```python
from build123d import *

# Parameters (mm, degrees)
SK_MAIN_EXTRUSION_R   = 3.4
SK_MAIN_EXTRUSION_R_2 = 9
MAIN_EXTRUSION_DEPTH  = 25


with BuildPart() as part:
    # Sk Main Extrusion → Main Extrusion (new body)
    with BuildSketch(Plane.XY):
        with BuildLine():
            Line((-35.964339765, 8.84120158), (-38.698942589, 10.116367819))
            ThreePointArc((-38.698942589, 10.116367819), (-39.146142418, 10.175242794), (-39.546236371, 9.966967065))
            Line((-39.546236371, 9.966967065), (-48.436814511, 1.076388924))
            ThreePointArc((-48.436814511, 1.076388924), (-48.876154339, 0.015728753), (-48.436814511, -1.044931419))
            Line((-48.436814511, -1.044931419), (-35.355339059, -14.126406871))
            ThreePointArc((-35.355339059, -14.126406871), (0, -28.771067812), (35.355339059, -14.126406871))
            Line((35.355339059, -14.126406871), (48.436814511, -1.044931419))
            ThreePointArc((48.436814511, -1.044931419), (48.876154339, 0.015728753), (48.436814511, 1.076388924))
            Line((48.436814511, 1.076388924), (39.546236371, 9.966967065))
            ThreePointArc((39.546236371, 9.966967065), (39.146142418, 10.175242794), (38.698942589, 10.116367819))
            Line((38.698942589, 10.116367819), (35.964339765, 8.84120158))
            ThreePointArc((35.964339765, 8.84120158), (35.87848322, 8.775321536), (35.828512874, 8.679329395))
            Line((35.828512874, 8.679329395), (35.425239457, 7.174292513))
            Line((35.425239457, 7.174292513), (35.753978107, 6.469310204))
            Line((35.753978107, 6.469310204), (38.336524222, 5.265049173))
            ThreePointArc((38.336524222, 5.265049173), (38.606308031, 4.948092133), (38.542703923, 4.53675336))
            ThreePointArc((38.542703923, 4.53675336), (36.486225813, 2.654969004), (33.783331243, 1.973371234))
            Line((33.783331243, 1.973371234), (32.420845917, 1.973371234))
            ThreePointArc((32.420845917, 1.973371234), (25.880108191, 4.682633508), (23.170845917, 11.223371234))
            Line((23.170845917, 11.223371234), (23.170845917, 12.585856559))
            ThreePointArc((23.170845917, 12.585856559), (23.852443688, 15.28875113), (25.734228043, 17.34522924))
            ThreePointArc((25.734228043, 17.34522924), (26.145566816, 17.408833348), (26.462523856, 17.139049539))
            Line((26.462523856, 17.139049539), (27.666784887, 14.556503424))
            Line((27.666784887, 14.556503424), (28.371767196, 14.227764774))
            Line((28.371767196, 14.227764774), (29.876804078, 14.631038191))
            ThreePointArc((29.876804078, 14.631038191), (29.972796219, 14.681008536), (30.038676264, 14.766865082))
            Line((30.038676264, 14.766865082), (31.313842502, 17.501467906))
            ThreePointArc((31.313842502, 17.501467906), (31.372717477, 17.948667735), (31.164441748, 18.348761688))
            Line((31.164441748, 18.348761688), (21.652543264, 27.860660172))
            ThreePointArc((21.652543264, 27.860660172), (21.165908241, 28.185819299), (20.591883092, 28.3))
            Line((20.591883092, 28.3), (5.926823816, 28.3))
            ThreePointArc((5.926823816, 28.3), (5.496641489, 28.164364033), (5.222054351, 27.806515107))
            Line((5.222054351, 27.806515107), (4.190076845, 24.971180212))
            ThreePointArc((4.190076845, 24.971180212), (4.175951325, 24.863886241), (4.208493649, 24.760675177))
            Line((4.208493649, 24.760675177), (4.987558066, 23.411296024))
            Line((4.987558066, 23.411296024), (5.718509166, 23.145251581))
            Line((5.718509166, 23.145251581), (8.396186179, 24.11984631))
            ThreePointArc((8.396186179, 24.11984631), (8.811074612, 24.086489799), (9.056960151, 23.750654467))
            ThreePointArc((9.056960151, 23.750654467), (8.933433013, 20.965882372), (7.504160339, 18.572684887))
            Line((7.504160339, 18.572684887), (6.540737726, 17.609262274))
            ThreePointArc((6.540737726, 17.609262274), (0, 14.9), (-6.540737726, 17.609262274))
            Line((-6.540737726, 17.609262274), (-7.504160339, 18.572684887))
            ThreePointArc((-7.504160339, 18.572684887), (-8.933433013, 20.965882372), (-9.056960151, 23.750654467))
            ThreePointArc((-9.056960151, 23.750654467), (-8.811074612, 24.086489799), (-8.396186179, 24.11984631))
            Line((-8.396186179, 24.11984631), (-5.718509166, 23.145251581))
            Line((-5.718509166, 23.145251581), (-4.987558066, 23.411296024))
            Line((-4.987558066, 23.411296024), (-4.208493649, 24.760675177))
            ThreePointArc((-4.208493649, 24.760675177), (-4.175951325, 24.863886241), (-4.190076845, 24.971180212))
            Line((-4.190076845, 24.971180212), (-5.222054351, 27.806515107))
            ThreePointArc((-5.222054351, 27.806515107), (-5.496641489, 28.164364033), (-5.926823816, 28.3))
            Line((-5.926823816, 28.3), (-20.591883092, 28.3))
            ThreePointArc((-20.591883092, 28.3), (-21.165908241, 28.185819299), (-21.652543264, 27.860660172))
            Line((-21.652543264, 27.860660172), (-31.164441748, 18.348761688))
            ThreePointArc((-31.164441748, 18.348761688), (-31.372717477, 17.948667735), (-31.313842502, 17.501467906))
            Line((-31.313842502, 17.501467906), (-30.038676264, 14.766865082))
            ThreePointArc((-30.038676264, 14.766865082), (-29.972796219, 14.681008536), (-29.876804078, 14.631038191))
            Line((-29.876804078, 14.631038191), (-28.371767196, 14.227764774))
            Line((-28.371767196, 14.227764774), (-27.666784887, 14.556503424))
            Line((-27.666784887, 14.556503424), (-26.462523856, 17.139049539))
            ThreePointArc((-26.462523856, 17.139049539), (-26.145566816, 17.408833348), (-25.734228043, 17.34522924))
            ThreePointArc((-25.734228043, 17.34522924), (-23.852443688, 15.28875113), (-23.170845917, 12.585856559))
            Line((-23.170845917, 12.585856559), (-23.170845917, 11.223371234))
            ThreePointArc((-23.170845917, 11.223371234), (-25.880108191, 4.682633508), (-32.420845917, 1.973371234))
            Line((-32.420845917, 1.973371234), (-33.783331243, 1.973371234))
            ThreePointArc((-33.783331243, 1.973371234), (-36.486225813, 2.654969004), (-38.542703923, 4.53675336))
            ThreePointArc((-38.542703923, 4.53675336), (-38.606308031, 4.948092133), (-38.336524222, 5.265049173))
            Line((-38.336524222, 5.265049173), (-35.753978107, 6.469310204))
            Line((-35.753978107, 6.469310204), (-35.425239457, 7.174292513))
            Line((-35.425239457, 7.174292513), (-35.828512874, 8.679329395))
            ThreePointArc((-35.828512874, 8.679329395), (-35.87848322, 8.775321536), (-35.964339765, 8.84120158))
        make_face()
        with Locations((0, -19.1)):
            Circle(SK_MAIN_EXTRUSION_R, mode=Mode.SUBTRACT)
        Circle(SK_MAIN_EXTRUSION_R_2, mode=Mode.SUBTRACT)
        with Locations((18.106601718, 20.8)):
            Circle(SK_MAIN_EXTRUSION_R, mode=Mode.SUBTRACT)
        with Locations((-18.106601718, 20.8)):
            Circle(SK_MAIN_EXTRUSION_R, mode=Mode.SUBTRACT)
        with BuildLine():
            Line((-33.410795411, -12.181863223), (-43.025551853, -2.567106781))
            ThreePointArc((-43.025551853, -2.567106781), (-43.242324604, -1.477316568), (-42.318445072, -0.86))
            Line((-42.318445072, -0.86), (-12.360841395, -0.86))
            ThreePointArc((-12.360841395, -0.86), (-11.708461138, -1.102108187), (-11.371974084, -1.7112))
            ThreePointArc((-11.371974084, -1.7112), (-8.980737669, -7.183059997), (-4.167977698, -10.718113729))
            ThreePointArc((-4.167977698, -10.718113729), (-2.911454942, -12.309920658), (-3.692145622, -14.181609948))
            ThreePointArc((-3.692145622, -14.181609948), (-6.052344462, -18.008383533), (-5.177787873, -22.418585955))
            ThreePointArc((-5.177787873, -22.418585955), (-5.184897798, -24.588029411), (-7.164897408, -25.474673081))
            ThreePointArc((-7.164897408, -25.474673081), (-21.348803489, -20.923067641), (-33.410795411, -12.181863223))
        make_face(mode=Mode.SUBTRACT)
        with BuildLine():
            Line((43.025551853, -2.567106781), (33.410795411, -12.181863223))
            ThreePointArc((33.410795411, -12.181863223), (21.348803489, -20.923067641), (7.164897408, -25.474673081))
            ThreePointArc((7.164897408, -25.474673081), (5.184897798, -24.588029411), (5.177787873, -22.418585955))
            ThreePointArc((5.177787873, -22.418585955), (6.052344462, -18.008383533), (3.692145622, -14.181609948))
            ThreePointArc((3.692145622, -14.181609948), (2.911454942, -12.309920658), (4.167977698, -10.718113729))
            ThreePointArc((4.167977698, -10.718113729), (8.980737669, -7.183059997), (11.371974084, -1.7112))
            ThreePointArc((11.371974084, -1.7112), (11.708461138, -1.102108187), (12.360841395, -0.86))
            Line((12.360841395, -0.86), (42.318445072, -0.86))
            ThreePointArc((42.318445072, -0.86), (43.242324604, -1.477316568), (43.025551853, -2.567106781))
        make_face(mode=Mode.SUBTRACT)
        with BuildLine():
            Line((22.313779306, 1.89), (12.161328052, 1.89))
            ThreePointArc((12.161328052, 1.89), (11.541328052, 2.10539819), (11.188421808, 2.6588))
            ThreePointArc((11.188421808, 2.6588), (8.576111126, 7.661613273), (3.898250872, 10.819133058))
            ThreePointArc((3.898250872, 10.819133058), (3.237253097, 11.766839243), (3.911288501, 12.70531745))
            ThreePointArc((3.911288501, 12.70531745), (7.825101881, 14.952320052), (10.632154811, 18.486072973))
            ThreePointArc((10.632154811, 18.486072973), (11.559727768, 19.021547306), (12.439624063, 18.410886302))
            ThreePointArc((12.439624063, 18.410886302), (15.272696143, 15.341842876), (19.412884455, 14.790330674))
            ThreePointArc((19.412884455, 14.790330674), (20.329585798, 14.523052251), (20.604120456, 13.608497808))
            ThreePointArc((20.604120456, 13.608497808), (20.697886834, 8.284715824), (23.085806686, 3.525589274))
            ThreePointArc((23.085806686, 3.525589274), (23.218099292, 2.463144798), (22.313779306, 1.89))
        make_face(mode=Mode.SUBTRACT)
        with BuildLine():
            Line((-12.161328052, 1.89), (-22.313779306, 1.89))
            ThreePointArc((-22.313779306, 1.89), (-23.218099292, 2.463144798), (-23.085806686, 3.525589274))
            ThreePointArc((-23.085806686, 3.525589274), (-20.697886834, 8.284715824), (-20.604120456, 13.608497808))
            ThreePointArc((-20.604120456, 13.608497808), (-20.329585798, 14.523052251), (-19.412884455, 14.790330674))
            ThreePointArc((-19.412884455, 14.790330674), (-15.272696143, 15.341842876), (-12.439624063, 18.410886302))
            ThreePointArc((-12.439624063, 18.410886302), (-11.559727768, 19.021547306), (-10.632154811, 18.486072973))
            ThreePointArc((-10.632154811, 18.486072973), (-7.825101881, 14.952320052), (-3.911288501, 12.70531745))
            ThreePointArc((-3.911288501, 12.70531745), (-3.237253097, 11.766839243), (-3.898250872, 10.819133058))
            ThreePointArc((-3.898250872, 10.819133058), (-8.576111126, 7.661613273), (-11.188421808, 2.6588))
            ThreePointArc((-11.188421808, 2.6588), (-11.541328052, 2.10539819), (-12.161328052, 1.89))
        make_face(mode=Mode.SUBTRACT)
    extrude(amount=-MAIN_EXTRUSION_DEPTH)


solid = part.part
```
Can you work these out from the model? Positions are in its coordinate system, mm. A direction names the side the tool comes from. Coordinates: 2 decimals unless noted, no trailing zeros. Loops run counter-clockwise (first coordinate to the right, second up) from the corner with the lowest first, then second, coordinate; pieces in that order, holes last. Notation, with made-up numbers: (29.5, 86) - (39.5, 86) arc R19 ccw to (39.5, 96) - close; hole circle Ø8 at (77.5, -30.75). An arc over 180 degrees is marked (long way). Answer as CSV lines item,"result". Start each with the question number.
1) I need wall thicknesses on line 1 (Y direction, x = 0, z = -11.25); line 2 (Y direction, x = -20, z = -9.5); line 3 (Y direction, x = 25, z = -13.25). Which ranges of each line are inside material? Lowest first, please. Write a range as from..to.
2) Which directions (+Z, -Z, +X, -X, +Y, -Y) give clear straight access to the entire face, cutting with the end or side of a thin tool? Please do faces 1 (the flat face through (-30.685, 16.153, -12.325)), 2 (the flat face through (4.713, 26.409, -12.325)), 3 (the cylindrical face through (15.22, 15.37, -12.32)).
3) Suppose I cut it at D-D (z = -8). Count the separate pieces of the cut face and the enclosed holes in it, plus the area to 3 significant figures.
4) For pin 1 (12 mm diameter, centred on x = -37.5, z = -18.5, fed in from -Y); pin 2 (0.7 mm diameter, centred on x = -33.5, z = -12.5, fed in from +Y); pin 3 (6 mm diameter, centred on x = 23.5, y = -4.5, fed in from +Z); pin 4 (10 mm diameter, centred on y = -12, z = -12, fed in from +X), each with a flat end and sliding along its axis, tell me the tip position at first contact or that it passes through.
5) Suppose I cut it at A-A (x = 0). Please give me the cut outline in (y, z), plus the area to 3 significant figures.
6) Thinking about a two-plate mould opening in X: for faces 4 (the flat face through (-4, 10, 0)), 5 (the flat face through (27, -0.86, -12)), 6 (the flat face through (30.67, 16.12, -12.32)), which applies, pulls with the +X half, pulls with the -X half, needs draft (parallel to the pull), parting line crosses it, or undercut?
7) Suppose I cut it at B-B (y = 20.8). Please give me the cut outline in (x, z), plus the area to 3 significant figures.
8) Suppose I cut it at C-C (x = 17.5). Please give me the cut outline in (y, z).
Check result:
1,line 1,"y = -28.77..-22.5, -15.7..-9, 9..14.9"
1,line 2,"y = -24.6..-21.58, -0.86..1.89, 14.74..17.98, 23.62..28.3"
1,line 3,"y = -22.07..-18.87, -0.86..5.7, 16.77..24.51"
2,face 1,"+Z, -Z, -X"
2,face 2,"+Z, -Z, +Y"
2,face 3,"+Z, -Z"
3,separate pieces,"1"
3,enclosed holes,"8"
3,area,"1,470 mm²"
4,pin 1,"stops at y = -17.6"
4,pin 2,"stops at y = 1.97"
4,pin 3,"passes through"
4,pin 4,"stops at x = 42.48"
5,outline,"(-28.77, -25) - (-22.5, -25) - (-22.5, 0) - (-28.77, 0) - close; (-15.7, -25) - (-9, -25) - (-9, 0) - (-15.7, 0) - close; (9, -25) - (14.9, -25) - (14.9, 0) - (9, 0) - close"
5,area,"472 mm²"
6,face 4,"needs draft"
6,face 5,"undercut"
6,face 6,"pulls with the +X half"
7,outline,"(-28.71, -25) - (-21.51, -25) - (-21.51, 0) - (-28.71, 0) - close; (-14.71, -25) - (-8.88, -25) - (-8.88, 0) - (-14.71, 0) - close; (8.88, -25) - (14.71, -25) - (14.71, 0) - (8.88, 0) - close; (21.51, -25) - (28.71, -25) - (28.71, 0) - (21.51, 0) - close"
7,area,"652 mm²"
8,outline,"(-25.61, -25) - (-22.66, -25) - (-22.66, 0) - (-25.61, 0) - close; (-0.86, -25) - (1.89, -25) - (1.89, 0) - (-0.86, 0) - close; (14.68, -25) - (17.45, -25) - (17.45, 0) - (14.68, 0) - close; (24.15, -25) - (28.3, -25) - (28.3, 0) - (24.15, 0) - close"
